Geometry check sheet. Reference: drawing and pictorial views, mm from the part's lowest x, y, z. A direction names the side the tool comes from. Round coordinates to 2 decimals unless told otherwise and drop trailing zeros. Write each loop counter-clockwise with the first axis right and the second up, starting at its lowest first coordinate (ties: lowest second). Pieces come first, ordered by that corner, then holes.
Item 1: Section check B-B, the plane x = 74.85. Record the cut outline in (y, z).
Item 2: Section check A-A, the plane z = 6.5. Record the cut outline in (x, y) (1 decimal), plus the area to 3 significant figures.
Item 3: Set-up check for the marked faces 1, 2 and 3: record each of +Z, -Z, +X, -X, +Y, -Y from which the full face is reachable in a straight line by a thin tool's end or side.
Item 4: Section check C-C, the plane z = 23.85. State how many separate pieces and enclosed holes the cut face has, plus the area to 3 significant figures.
Item 5: Depth check by flat-ended pin: pin 1 (9 mm diameter, centred on y = 75, z = 18.5, fed in from -X); pin 2 (6.5 mm diameter, centred on x = 79.5, y = 76, fed in from -Z); pin 3 (1 mm diameter, centred on x = 51, z = 36, fed in from -Y); pin 4 (4 mm diameter, centred on y = 74, z = 33.5, fed in from +X). Enter the tip coordinate at first touch or a pass-through.
Item 6: Material ranges on line 1 along X through (y, z) = (76.5, 23.85); line 2 along Z through (x, y) = (74.85, 77); line 3 along Y through (x, z) = (139.5, 29), recorded low to high.
Item 7: Section check D-D, the plane x = 128. Record the cut outline in (y, z).
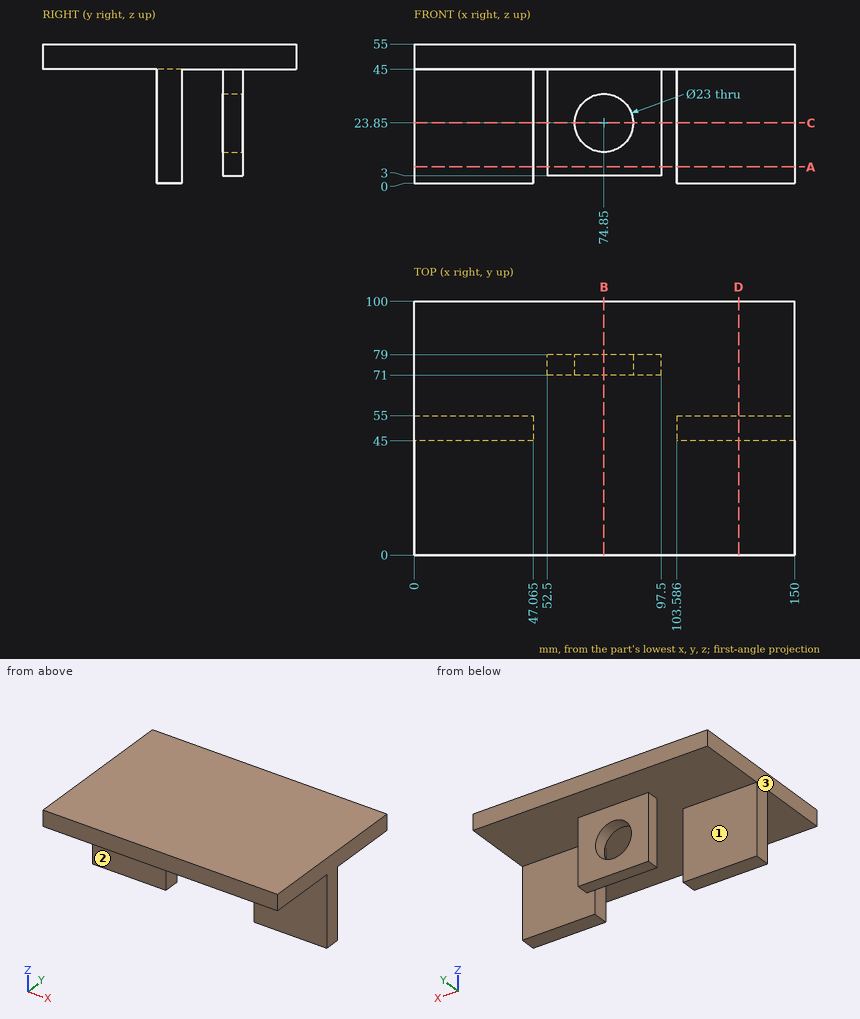
Values found:
1. outline: (0, 45) - (71, 45) - (71, 35.35) - (79, 35.35) - (79, 45) - (100, 45) - (100, 55) - (0, 55) - close; (71, 3) - (79, 3) - (79, 12.35) - (71, 12.35) - close
2. outline: (0, 45) - (47.1, 45) - (47.1, 55) - (0, 55) - close; (52.5, 71) - (97.5, 71) - (97.5, 79) - (52.5, 79) - close; (103.6, 45) - (150, 45) - (150, 55) - (103.6, 55) - close
2. area: 1,290 mm2
3. face 1: -Z, +X, -X, +Y
3. face 2: -Z, +X, -X, -Y
3. face 3: +Z, -Z, -X, +Y, -Y
4. separate pieces: 4
4. enclosed holes: 0
4. area: 1,110 mm2
5. pin 1: stops at x = 52.5
5. pin 2: stops at z = 3
5. pin 3: passes through
5. pin 4: stops at x = 97.5
6. line 1: x = 52.5 to 63.35, 86.35 to 97.5
6. line 2: z = 3 to 12.35, 35.35 to 55
6. line 3: y = 45 to 55
7. outline: (0, 45) - (45, 45) - (45, 0) - (55, 0) - (55, 45) - (100, 45) - (100, 55) - (0, 55) - close
